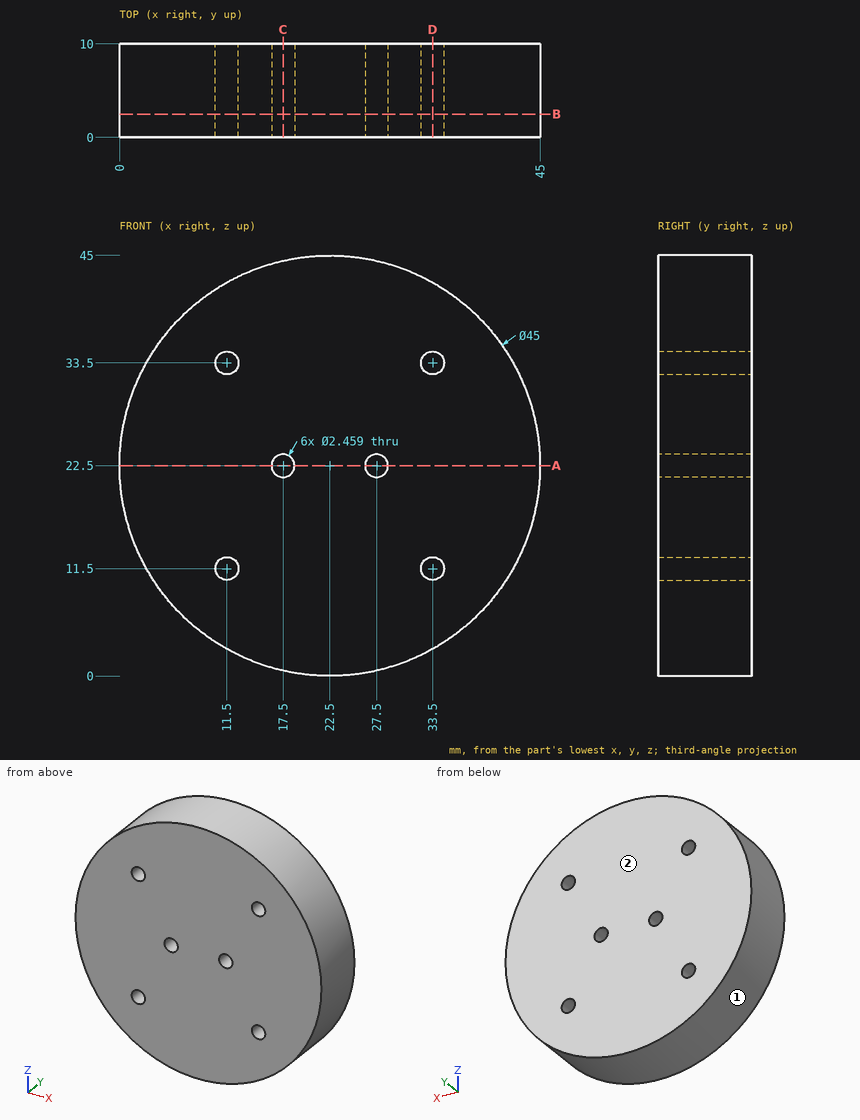
Can you work these out from the drawing? Everything is in mm from the part's minimum corner. Round coordinates to 2 decimals unless told otherwise and drop trailing zeros. Write each loop counter-clockwise with the first axis right and the second up, starting at its lowest first coordinate (ties: lowest second). Pieces come first, ordered by that corner, then holes. Notation, with made-up numbers: (41, 38.25) - (100, 38.25) arc R19 cw to (100, 53.25) - close; hole circle Ø1 at (2.25, 82.25). An arc over 180 degrees is marked (long way). Use a Markdown table: item, result.
Q1. For pin 1 (1.5 mm diameter, centred on y = 4.5, z = 37, fed in from -X); pin 2 (5 mm diameter, centred on y = 8.5, z = 6, fed in from +X); pin 3 (1 mm diameter, centred on y = 2.5, z = 15.5, fed in from -X), each with a flat end and sliding along its axis, tell me the tip position at first contact or that it passes through.
Output values:
| item | result |
|---|---|
| pin 1 | x = 4.69 |
| pin 2 | x = 40.11 |
| pin 3 | x = 0.96 |
Q2. I want a section at D-D (x = 33.5). List the corners of the cut face in (y, z) for me.
Output values:
| item | result |
|---|---|
| outline | (0, 2.87) - (10, 2.87) - (10, 10.27) - (0, 10.27) - close; (0, 12.73) - (10, 12.73) - (10, 32.27) - (0, 32.27) - close; (0, 34.73) - (10, 34.73) - (10, 42.13) - (0, 42.13) - close |
Q3. I want a section at B-B (y = 2.5). List the corners of the cut face in (x, z) for me.
Output values:
| item | result |
|---|---|
| outline | circle Ø45 at (22.5, 22.5); hole circle Ø2.46 at (11.5, 11.5); hole circle Ø2.46 at (11.5, 33.5); hole circle Ø2.46 at (17.5, 22.5); hole circle Ø2.46 at (27.5, 22.5); hole circle Ø2.46 at (33.5, 11.5); hole circle Ø2.46 at (33.5, 33.5) |
Q4. I want a section at A-A (z = 22.5). List the corners of the cut face in (x, y) for me.
Output values:
| item | result |
|---|---|
| outline | (0, 0) - (16.27, 0) - (16.27, 10) - (0, 10) - close; (18.73, 0) - (26.27, 0) - (26.27, 10) - (18.73, 10) - close; (28.73, 0) - (45, 0) - (45, 10) - (28.73, 10) - close |
Q5. Thinking about a two-plate mould opening in Z: for the marked faces 1 and 2, which applies, released by +Z, released by -Z, zero draft, split by the parting line, or undercut?
Output values:
| item | result |
|---|---|
| face 1 | split by the parting line |
| face 2 | zero draft |
Q6. Please list where these lines run through material, in increasing order: L1, parallel to X at y = 1.25, z = 33; L2, parallel to X at y = 3, z = 33.5.
Output values:
| item | result |
|---|---|
| L1 | 2.6 to 10.38, 12.62 to 32.38, 34.62 to 42.4 |
| L2 | 2.87 to 10.27, 12.73 to 32.27, 34.73 to 42.13 |
Q7. I want a section at C-C (x = 17.5). List the corners of the cut face in (y, z) for me.
Output values:
| item | result |
|---|---|
| outline | (0, 0.56) - (10, 0.56) - (10, 21.27) - (0, 21.27) - close; (0, 23.73) - (10, 23.73) - (10, 44.44) - (0, 44.44) - close |
